Study the drawing (mm; zero at the part's minimum x, y, z) and answer. Coordinates: 2 decimals unless noted, no trailing zeros. Write each loop counter-clockwise with the first axis right and the second up, starting at its lowest first coordinate (ties: lowest second). Pieces come first, ordered by that corner, then holes. Notation, with made-up numbers: (60, 40) -> (88, 40) arc R11 cw to (88, 61) -> close; hole circle Ø7 at (9, 82.5). An arc over 180 degrees is marked (long way). Answer in a Markdown table with one row per item. Add a question column.
Item 1: Section B-B on y = 36 is taken. Write down the section's boundary in (x, z).
Item 2: Section D-D on y = 22 is taken. Write down the section's boundary in (x, z) (1 decimal), then the cut area to 3 significant figures.
Item 3: Section C-C on z = 27.5 is taken. Write down the section's boundary in (x, y).
Item 4: Section A-A on x = 1.3 is taken. Write down the section's boundary in (y, z), then the cut area to 3 significant figures.
Item 5: Straight lines are drawn through the part: line 1 (Y direction, x = 2.1, z = 27.5); line 2 (Y direction, x = 1.35, z = 12) (1 decimal); line 3 (Z direction, x = 0.5, y = 33.5) (1 decimal). For each, find the intervals that lie inside material, in ascending order. Write a range as from..to.
Item 6: Given pin 1 Ø1.9 at (y, z) = (36, 42.22) entering from -X (1 decimal); pin 2 Ø1.5 at (x, y) = (1, 6) entering from +Z (1 decimal); pin 3 Ø1 at (x, z) = (0.5, 19) entering from +Y; pin 4 Ø1.5 at (x, y) = (2.5, 26) entering from +Z, each flat-ended and moving along its own axis, determine where each tip first touches the part or whether it passes through.
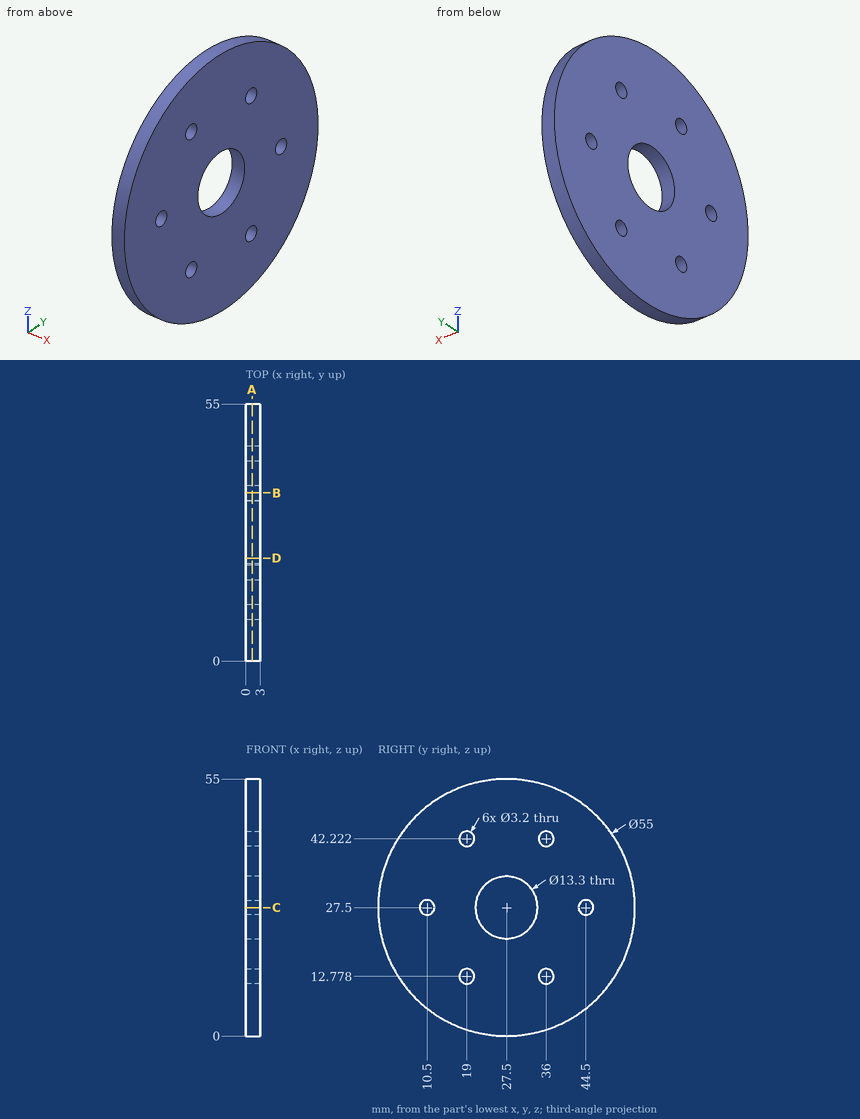
Results below:
| question | item | result |
|---|---|---|
| 1 | outline | (0, 1.35) -> (3, 1.35) -> (3, 11.18) -> (0, 11.18) -> close; (0, 14.38) -> (3, 14.38) -> (3, 40.62) -> (0, 40.62) -> close; (0, 43.82) -> (3, 43.82) -> (3, 53.65) -> (0, 53.65) -> close |
| 2 | outline | (0, 0.6) -> (3, 0.6) -> (3, 23.8) -> (0, 23.8) -> close; (0, 31.2) -> (3, 31.2) -> (3, 54.4) -> (0, 54.4) -> close |
| 2 | area | 139 mm2 |
| 3 | outline | (0, 0) -> (3, 0) -> (3, 8.9) -> (0, 8.9) -> close; (0, 12.1) -> (3, 12.1) -> (3, 20.85) -> (0, 20.85) -> close; (0, 34.15) -> (3, 34.15) -> (3, 42.9) -> (0, 42.9) -> close; (0, 46.1) -> (3, 46.1) -> (3, 55) -> (0, 55) -> close |
| 4 | outline | circle Ø55 at (27.5, 27.5); hole circle Ø3.2 at (10.5, 27.5); hole circle Ø3.2 at (19, 12.78); hole circle Ø3.2 at (19, 42.22); hole circle Ø13.3 at (27.5, 27.5); hole circle Ø3.2 at (36, 12.78); hole circle Ø3.2 at (36, 42.22); hole circle Ø3.2 at (44.5, 27.5) |
| 4 | area | 2,190 mm2 |
| 5 | line 1 | y = 0..8.9, 12.1..20.85, 34.15..42.9, 46.1..55 |
| 5 | line 2 | y = 4.8..17.6, 20.4..34.6, 37.4..50.2 |
| 5 | line 3 | z = 0.7..24.6, 30.4..54.3 |
| 6 | pin 1 | passes through |
| 6 | pin 2 | stops at z = 45.5 |
| 6 | pin 3 | stops at y = 53.81 |
| 6 | pin 4 | stops at z = 54.99 |
